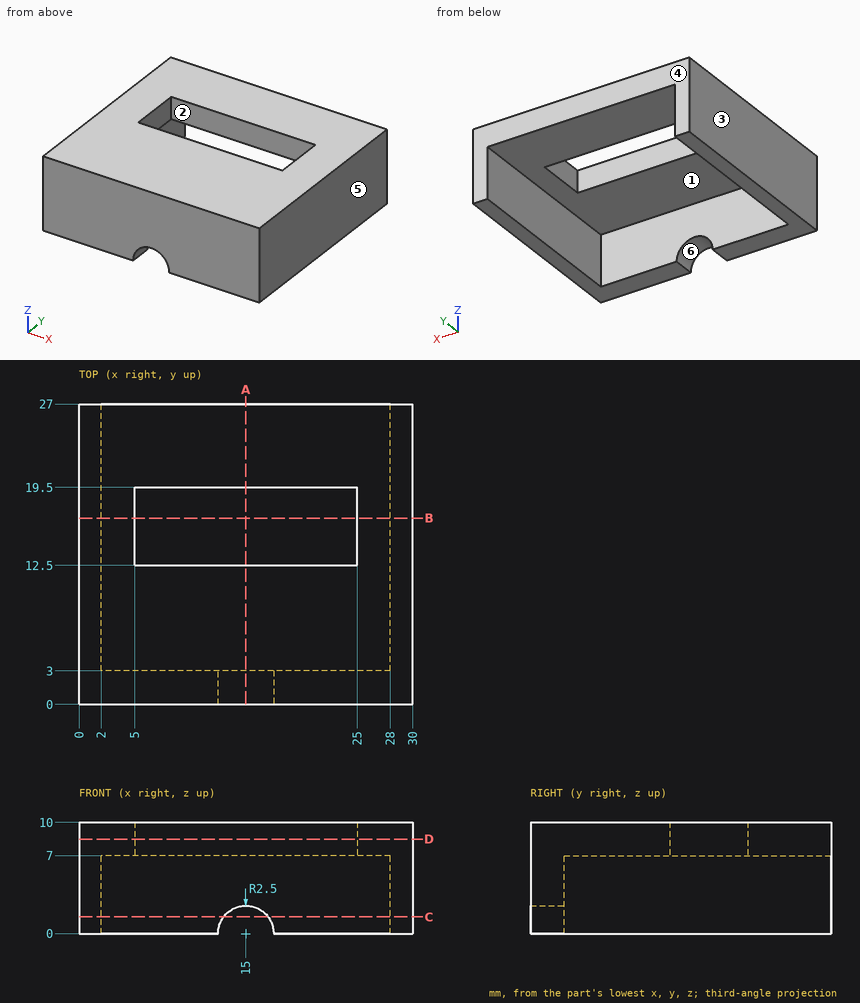
Could you check a few things on this drawing? It's one solid part, dimensions in mm from its lowest x, y, z. A direction names the side the tool comes from. Give positions to 0.01 mm unless a question says otherwise; leave off trailing zeros. Order: outer loops, then holes, each group sorted by start corner. A loop starts at its lowest first (then second) coordinate and runs counter-clockwise, first axis right, second up. Notation, with made-up numbers: (8, 74) -> (45, 74) arc R9 ccw to (45, 83) -> close; hole circle Ø2 at (37, -6). An arc over 180 degrees is marked (long way). Use CSV: the item, a comma, the result in double quotes. Start each with the question number.
Item 1: Suppose I cut it at D-D (z = 8.5). List the corners of the cut face in (x, y) for me, and give its area (3 significant figures).
Item 2: If I drill on probe 1 along X at (y, z) = (23, 1.25); probe 2 along Y at (x, z) = (9.5, 8.75); probe 3 along X at (y, z) = (14, 8), over which ranges is the centre line in solid material (lowest first)? Write a range as [from, to].
Item 3: On a 3-axis mill with a long thin cutter (end or side, diameter ignored), from which of +Z, -Z, +X, -X, +Y, -Y can I reach the whole of each face in a straight line? I mean the marked faces 1, 2 and 3. Say none if no direction works.
Item 4: Thinking about a two-plate mould opening in X: for the marked faces 4, 5 and 6, which applies, pulls with the +X half, pulls with the -X half, needs draft (parallel to the pull), parting line crosses it, or undercut?
Item 5: Suppose I cut it at B-B (y = 16.75). List the corners of the cut face in (x, z) for me, and give its area (3 significant figures).
Item 6: I'm going to push flat-ended pins straight in: P1, Ø3.5, axis at x = 15.5, z = 2.5, coming from the +Y side; P2, Ø3, axis at x = 12, y = 21.5, coming from the -Z side. Where does each tip first touch, or does it pass through?
Item 7: Suppose I cut it at C-C (z = 1.5). List the corners of the cut face in (x, y) for me.
Item 8: Suppose I cut it at A-A (x = 15). List the corners of the cut face in (y, z) for me.
Answer block:
1,outline,"(0, 0) -> (30, 0) -> (30, 27) -> (0, 27) -> close; hole (5, 12.5) -> (25, 12.5) -> (25, 19.5) -> (5, 19.5) -> close"
1,area,"670 mm^2"
2,probe 1,"x = [0, 2], [28, 30]"
2,probe 2,"y = [0, 12.5], [19.5, 27]"
2,probe 3,"x = [0, 5], [25, 30]"
3,face 1,"-Z, +Y"
3,face 2,"+Z, -Z"
3,face 3,"+Z, -Z, -X, +Y, -Y"
4,face 4,"needs draft"
4,face 5,"pulls with the +X half"
4,face 6,"undercut"
5,outline,"(0, 0) -> (2, 0) -> (2, 7) -> (5, 7) -> (5, 10) -> (0, 10) -> close; (25, 7) -> (28, 7) -> (28, 0) -> (30, 0) -> (30, 10) -> (25, 10) -> close"
5,area,"58.0 mm^2"
6,P1,"stops at y = 3"
6,P2,"stops at z = 7"
7,outline,"(0, 0) -> (13, 0) -> (13, 3) -> (2, 3) -> (2, 27) -> (0, 27) -> close; (17, 0) -> (30, 0) -> (30, 27) -> (28, 27) -> (28, 3) -> (17, 3) -> close"
8,outline,"(0, 2.5) -> (3, 2.5) -> (3, 7) -> (12.5, 7) -> (12.5, 10) -> (0, 10) -> close; (19.5, 7) -> (27, 7) -> (27, 10) -> (19.5, 10) -> close"
